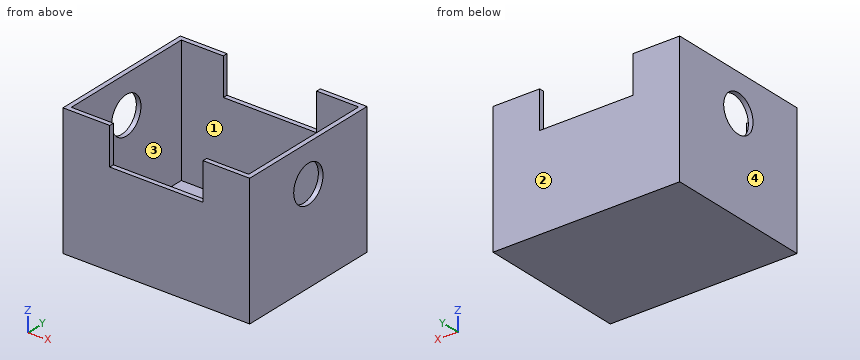
from build123d import *

# Parameters (mm, degrees)
F0_W     = 100
F0_H     = 80
F1_DEPTH = 70
F2_T     = -2.5
F3_W     = 50
F3_H     = 20
F4_DEPTH = 80.001
F5_R     = 10
F6_DEPTH = 100.001


with BuildPart() as f1:
    # F0 (on Top) → F1 (new body)
    with BuildSketch(Plane.XY):
        Rectangle(F0_W, F0_H)
    extrude(amount=F1_DEPTH)

    # F2
    f2_openings = [f1.faces().sort_by_distance(p)[0] for p in [
        (0, 0, 70),
    ]]
    offset(amount=F2_T, openings=f2_openings)

    # F3 (on face) → F4 (cut, through all)
    with BuildSketch(Plane.XZ.offset(40)):
        with Locations((0, 60)):
            Rectangle(F3_W, F3_H)
    extrude(amount=-F4_DEPTH, mode=Mode.SUBTRACT)

    # F5 (on face) → F6 (cut, through all)
    with BuildSketch(Plane(origin=(-50, 0, 0), x_dir=(0, -1, 0), z_dir=(-1, 0, 0))):
        with Locations((0, 50)):
            Circle(F5_R)
    extrude(amount=-F6_DEPTH, mode=Mode.SUBTRACT)


solid = f1.part
The listing builds one solid part. Answer for the finished solid, in the listing's coordinates (mm). Face numbers are marked on the shaded views. Round coordinates to 2 decimals unless told otherwise and drop trailing zeros. Order: outer loops, then holes, each group sorted by start corner. A loop starts at its lowest first (then second) coordinate and runs counter-clockwise, first axis right, second up. Notation, with made-up numbers: (80, 16) -> (120, 16) arc R16 ccw to (120, 23) -> close; hole circle Ø6 at (19.25, 74.25). An arc over 180 degrees is marked (long way). One line per item, written item: value.
Item 1: Find section B-B, the plane y = 0. Give the vertices of the cut face in (x, z), then the cut area to 4 significant figures.
Taken from the geometry:
outline: (-50, 0) -> (50, 0) -> (50, 40) -> (47.5, 40) -> (47.5, 2.5) -> (-47.5, 2.5) -> (-47.5, 40) -> (-50, 40) -> close; (-50, 60) -> (-47.5, 60) -> (-47.5, 70) -> (-50, 70) -> close; (47.5, 60) -> (50, 60) -> (50, 70) -> (47.5, 70) -> close
area: 487.5 mm2
Item 2: Given P1, Ø3, axis at x = 27, y = -1, coming from the +Z side; P2, Ø1.5, axis at x = -6.5, y = -5, coming from the -Z side; P3, Ø0.8, axis at x = 6, y = 38.5, coming from the +Z side, each flat-ended and moving along its own axis, determine where each tip first touches the part or whether it passes through.
Taken from the geometry:
P1: stops at z = 2.5
P2: stops at z = 0
P3: stops at z = 50
Item 3: Find section A-A, the plane x = -18.5. Give the vertices of the cut face in (y, z).
Taken from the geometry:
outline: (-40, 0) -> (40, 0) -> (40, 50) -> (37.5, 50) -> (37.5, 2.5) -> (-37.5, 2.5) -> (-37.5, 50) -> (-40, 50) -> close
Item 4: Find section C-C, the plane z = 30. Give the vertices of the cut face in (x, y), then the cut area to 3 significant figures.
Taken from the geometry:
outline: (-50, -40) -> (50, -40) -> (50, 40) -> (-50, 40) -> close; hole (-47.5, -37.5) -> (47.5, -37.5) -> (47.5, 37.5) -> (-47.5, 37.5) -> close
area: 875 mm2
Item 5: For a pull along Y with two mould halves and no side action, classify the marked faces 1, 2, 3 and 4 as released by +Y, released by -Y, zero draft, split by the parting line, or undercut.
Taken from the geometry:
face 1: undercut
face 2: released by +Y
face 3: undercut
face 4: zero draft
Item 6: Straight lines are drawn through the part: L1, parallel to Z at x = -48, y = 0; L2, parallel to X at y = 8.5, z = 61.5; L3, parallel to Y at x = -17, z = 31. For each, find the intervals that lie inside material, in ascending order.
Taken from the geometry:
L1: z = 0 to 40, 60 to 70
L2: x = -50 to -47.5, 47.5 to 50
L3: y = -40 to -37.5, 37.5 to 40
Item 7: Find section D-D, the plane z = 45.5. Give the vertices of the cut face in (x, y), then the cut area to 3 significant figures.
Taken from the geometry:
outline: (-50, -40) -> (50, -40) -> (50, -8.93) -> (47.5, -8.93) -> (47.5, -37.5) -> (-47.5, -37.5) -> (-47.5, -8.93) -> (-50, -8.93) -> close; (-50, 8.93) -> (-47.5, 8.93) -> (-47.5, 37.5) -> (47.5, 37.5) -> (47.5, 8.93) -> (50, 8.93) -> (50, 40) -> (-50, 40) -> close
area: 786 mm2
